Read the model definition and answer for the solid it produces. Units are mm, in the model's axes. Face numbers are marked on the shaded views. A direction names the side the tool comes from. Coordinates: 2 decimals unless noted, no trailing zeros. Order: outer loops, then holes, each group sorted by start corner. A loop starts at its lowest first (then second) coordinate and runs counter-clockwise, first axis right, second up. Notation, with made-up numbers: (83, 4.5) -> (124, 4.5) arc R20 cw to (124, 22.5) -> close; hole circle Ø6 at (72.25, 46.25). An arc over 180 degrees is marked (long way). Answer in a Markdown table with one row per item.
Autodesk Inventor part; units mm, degrees
ref_plane "YZ Plane" through (0, 0, 0) normal (1, 0, 0) x (0, 1, 0)
ref_plane "XZ Plane" through (0, 0, 0) normal (0, 1, 0) x (-1, 0, 0)
ref_plane "XY Plane" through (0, 0, 0) normal (0, 0, 1) x (1, 0, 0)
sketch "Sketch12" plane through (0, 0, 0) normal (0, 0, 1) x (1, 0, 0)
  line L0 (0, 0) -> (35, 0)
  line L1 (35, 0) -> (35, 47)
  line L2 (35, 47) -> (0, 47)
  line L3 (0, 47) -> (0, 0)
  dimension "d49" = 35
  dimension "d50" = 47
extrude "Plate4" add sketch "Sketch12" along normal blind 1
sketch "Sketch13" plane through (0, 0, 0) normal (-1, 0, 0) x (0, 0, 1)
  point P0 (0, 0)
sketch "Sketch14" plane through (0, 46, 0) normal (0, 1, 0) x (-1, 0, 0)
  line L0 (-35, 0) -> (0, 0)
  line L1 (0, 0) -> (0, 12)
  line L2 (0, 12) -> (-35, 12)
  line L3 (-35, 12) -> (-35, 0)
edge flange "Flange3" height 12 angle 90 thickness 1 bend radius 1 thickness toward (0, 1, 0) relief tear relief width 1 relief depth 0.5 edges at (17.5, 47, 1) wall of the first edge with corners at (35, 46, 0) (0, 46, 0) (0, 46, 12) (35, 46, 12)
bend "Bend3"
corner "Corner3"
sketch "Sketch15" plane through (35, 1, 0) normal (0, -1, 0) x (1, 0, 0)
  line L0 (-35, 0) -> (0, 0)
  line L1 (0, 0) -> (0, 12)
  line L2 (0, 12) -> (-35, 12)
  line L3 (-35, 12) -> (-35, 0)
edge flange "Flange4" height 12 angle 90 thickness 1 bend radius 1 thickness toward (0, -1, 0) relief tear relief width 1 relief depth 0.5 edges at (17.5, 0, 1) wall of the first edge with corners at (0, 1, 0) (35, 1, 0) (35, 1, 12) (0, 1, 12)
bend "Bend4"
corner "Corner4"
sketch "Sketch16" plane through (0, 47, 12) normal (0, 1, 0) x (1, 0, 0)
  line L0 (0, 11) -> (0, 10)
  line L1 (0, 10) -> (0, 5.52) construction
  line L2 (0, 10) -> (0, 0)
  line L3 (0, 5.52) -> (9.5, 5.52) construction
  circle A0 centre (9.5, 5.52) radius 1.5
  line L4 (35, 10) -> (35, 0)
  line L5 (35, 10) -> (35, 5.52)
  line L6 (35, 5.52) -> (25.5, 5.52) construction
  circle A1 centre (25.5, 5.52) radius 1.5
  point P0 (0, 12)
  dimension "d72" = 4.48
  dimension "d73" = 9.5
  dimension "d74" = 3
  dimension "d75" = 4.48
  dimension "d76" = 9.5
  dimension "d77" = 3
extrude "Extrusion4" cut sketch "Sketch16" against normal through all
sketch "Sketch17" plane through (0, 0, 1) normal (0, 0, 1) x (1, 0, 0)
  line L0 (35, 45) -> (0, 45) construction
  line L1 (0, 45) -> (2, 45) construction
  line L2 (2, 45) -> (2, 35.5) construction
  line L3 (35, 45) -> (33, 45) construction
  line L4 (33, 45) -> (33, 35.5) construction
  circle A0 centre (2, 35.5) radius 1.25
  circle A1 centre (33, 35.5) radius 1.25
  point P0 (0, 0)
  dimension "d80" = 2
  dimension "d81" = 9.5
  dimension "d82" = 2
  dimension "d83" = 2.5
  dimension "d84" = 9.5
extrude "Extrusion5" cut sketch "Sketch17" against normal blind 10
sketch "Sketch18" plane through (0, 0, 1) normal (0, 0, 1) x (1, 0, 0)
  line L0 (0, 2) -> (0, 45)
  line L1 (0, 2) -> (6.5, 2) construction
  line L2 (6.5, 2) -> (6.5, 2.58) construction
  circle A0 centre (6.5, 2.58) radius 1.25
  line L3 (35, 45) -> (35, 2)
  line L4 (35, 2) -> (28.5, 2) construction
  line L5 (35, 2) -> (0, 2)
  line L6 (28.5, 2) -> (28.5, 2.58) construction
  circle A1 centre (28.5, 2.58) radius 1.25
  point P0 (0, 0)
  dimension "d87" = 6.5
  dimension "d88" = 0.58
  dimension "d89" = 2.5
  dimension "d90" = 6.5
  dimension "d91" = 0.58
  dimension "d92" = 2.5
extrude "Extrusion6" cut sketch "Sketch18" against normal blind 10
sketch "Sketch20" plane through (0, 0, 1) normal (0, 0, 1) x (1, 0, 0)
  arc A0 (7.6073, 2) -> (5.3927, 2) centre (6.5, 2.58) ccw
  arc A1 (5.3927, 2) -> (7.6073, 2) centre (6.5, 2.58) ccw
  circle A2 centre (6.5, 2.58) radius 1.25
  arc A3 (29.6073, 2) -> (27.3927, 2) centre (28.5, 2.58) ccw
  arc A4 (27.3927, 2) -> (29.6073, 2) centre (28.5, 2.58) ccw
  circle A5 centre (28.5, 2.58) radius 1.25
  point P0 (0, 0)
extrude "Extrusion7" cut sketch "Sketch20" along normal through all
equation "\"d51\" = Thickness"
equation "\"d52\" = BendReliefWidth"
equation "\"d53\" = BendReliefDepth"
equation "\"d54\" = MinimumRemnant"
equation "\"d55\" = TransitionRadius"
equation "\"d58\" = BendRadius"
equation "\"d59\" = CornerReliefSize"
equation "\"d60\" = GapSize"
equation "\"d61\" = JacobiRadiusSize"
equation "\"d62\" = BendReliefWidth"
equation "\"d63\" = BendReliefDepth"
equation "\"d64\" = MinimumRemnant"
equation "\"d65\" = TransitionRadius"
equation "\"d68\" = BendRadius"
equation "\"d69\" = CornerReliefSize"
equation "\"d70\" = GapSize"
equation "\"d71\" = JacobiRadiusSize"
equation "\"BendRadius\" = Thickness"
equation "\"BendReliefWidth\" = Thickness"
equation "\"BendReliefDepth\" = 0.5 * Thickness"
equation "\"CornerReliefSize\" = 4 * Thickness"
equation "\"MinimumRemnant\" = 2 * Thickness"
equation "\"TransitionRadius\" = BendRadius"
equation "\"JacobiRadiusSize\" = BendRadius"
equation "\"GapSize\" = Thickness"
properties part number "Suportmotor"
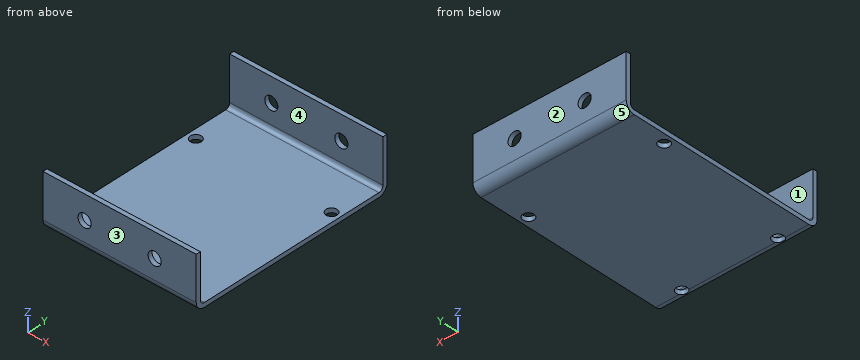
Q1. Given pin 1 (1.5 mm diameter, centred on x = 15, y = 9, fed in from +Z), flat-ended and moving along its own axis, determine where the tip first touches the part or whether it passes through.
Outcome:
| item | result |
|---|---|
| pin 1 | z = 1 |
Q2. The part is cut by section A-A (y = 35.5). Write down the section's boundary in (x, z).
Outcome:
| item | result |
|---|---|
| outline | (0, 0) -> (0.75, 0) -> (0.75, 1) -> (0, 1) -> close; (3.25, 0) -> (31.75, 0) -> (31.75, 1) -> (3.25, 1) -> close; (34.25, 0) -> (35, 0) -> (35, 1) -> (34.25, 1) -> close |
Q3. Consider line 1 (X direction, y = 2.58, z = 0.5); line 2 (Y direction, x = 12.5, z = 3.5); line 3 (Z direction, x = 29, y = 43). Determine where each line is inside the solid, lowest interval first.
Outcome:
| item | result |
|---|---|
| line 1 | 0 to 5.25, 7.75 to 27.25, 29.75 to 35 |
| line 2 | 0 to 1, 46 to 47 |
| line 3 | 0 to 1 |
Q4. The part is cut by section C-C (z = 10.5). Write down the section's boundary in (x, y).
Outcome:
| item | result |
|---|---|
| outline | (0, 0) -> (35, 0) -> (35, 1) -> (0, 1) -> close; (0, 46) -> (35, 46) -> (35, 47) -> (0, 47) -> close |
Q5. For the marked faces 4 and 5, determine the directions among +Z, -Z, +X, -X, +Y, -Y from which every point of the face is accessible in a straight line to the end or side of a thin tool.
Outcome:
| item | result |
|---|---|
| face 4 | +Z, +X, -X |
| face 5 | -Z, +X, -X, +Y |
Q6. For a pull along Y with two mould halves and no side action, classify the marked faces 1, 2 and 3 as pulls with the +Y half, pulls with the -Y half, needs draft (parallel to the pull), parting line crosses it, or undercut.
Outcome:
| item | result |
|---|---|
| face 1 | undercut |
| face 2 | pulls with the +Y half |
| face 3 | pulls with the -Y half |
Q7. The part is cut by section D-D (x = 12.5). Write down the section's boundary in (y, z), then the cut area to 3 significant figures.
Outcome:
| item | result |
|---|---|
| outline | (0, 2) arc R2 ccw to (2, 0) -> (45, 0) arc R2 ccw to (47, 2) -> (47, 12) -> (46, 12) -> (46, 2) arc R1 cw to (45, 1) -> (2, 1) arc R1 cw to (1, 2) -> (1, 12) -> (0, 12) -> close |
| area | 67.7 mm² |
Q8. The part is cut by section B-B (x = 25.5). Write down the section's boundary in (y, z), then the cut area to 3 significant figures.
Outcome:
| item | result |
|---|---|
| outline | (0, 2) arc R2 ccw to (2, 0) -> (45, 0) arc R2 ccw to (47, 2) -> (47, 4.98) -> (46, 4.98) -> (46, 2) arc R1 cw to (45, 1) -> (2, 1) arc R1 cw to (1, 2) -> (1, 4.98) -> (0, 4.98) -> close; (0, 7.98) -> (1, 7.98) -> (1, 12) -> (0, 12) -> close; (46, 7.98) -> (47, 7.98) -> (47, 12) -> (46, 12) -> close |
| area | 61.7 mm² |
